The listing builds one solid part. Answer for the finished solid, in the listing's coordinates (mm). A direction names the side the tool comes from. Coordinates: 2 decimals unless noted, no trailing zeros. Loops run counter-clockwise (first coordinate to the right, second up) from the corner with the lowest first, then second, coordinate; pieces in that order, holes last. Notation, with made-up numbers: (56, 4) - (97, 4) arc R16 cw to (97, 25) - close; hole circle Ø5 at (37, -11.5). An arc over 180 degrees is marked (long way). Put each result on its own line as item: value.
```python
from build123d import *

# Parameters (mm, degrees)
SKETCH1_W                      = 150
SKETCH1_H                      = 26
BOSS_EXTRUDE1_DEPTH            = 8
SKETCH2_R                      = 1
CUT_EXTRUDE1_DEPTH             = 10
SKETCH3_R                      = 1
CUT_EXTRUDE2_DEPTH             = 10
SKETCH4_W                      = 65
SKETCH4_H                      = 30
BOSS_EXTRUDE2_DEPTH            = 8
FILLET1_R                      = 32
SKETCH5_W                      = 70
SKETCH5_H                      = 30
BOSS_EXTRUDE3_DEPTH            = 8
CBORE_FOR_M4_SHCS1_D           = 4.5
CBORE_FOR_M4_SHCS1_CBORE_D     = 8
CBORE_FOR_M4_SHCS1_CBORE_DEPTH = 4
SKETCH10_W                     = 18
SKETCH10_H                     = 17
BOSS_EXTRUDE4_DEPTH            = 8
FILLET2_R                      = 10
FILLET3_R                      = 2
FILLET4_R                      = 4
SKETCH11_R                     = 1.6
CUT_EXTRUDE3_DEPTH             = 82.172655494
CUT_EXTRUDE5_START             = -5.2
CUT_EXTRUDE5_DEPTH             = 2.4


with BuildPart() as part:
    # Sketch1 → Boss-Extrude1 (new body)
    with BuildSketch(Plane(origin=(0, 0, 0), x_dir=(1, 0, 0), z_dir=(0, 1, 0))):
        Rectangle(SKETCH1_W, SKETCH1_H)
    extrude(amount=BOSS_EXTRUDE1_DEPTH)

    # Sketch2 → Cut-Extrude1 (cut)
    with BuildSketch(Plane(origin=(0, 0, -13), x_dir=(-1, 0, 0), z_dir=(0, 0, -1))):
        with Locations((47.4, 3.5)):
            Circle(SKETCH2_R)
        with Locations((-49.4, 3.5)):
            Circle(SKETCH2_R)
    extrude(amount=-CUT_EXTRUDE1_DEPTH, mode=Mode.SUBTRACT)

    # Sketch3 → Cut-Extrude2 (cut)
    with BuildSketch(Plane.XY.offset(13)):
        with Locations((1, 3.5)):
            Circle(SKETCH3_R)
    extrude(amount=-CUT_EXTRUDE2_DEPTH, mode=Mode.SUBTRACT)

    # Sketch4 → Boss-Extrude2 (add)
    with BuildSketch(Plane(origin=(0, 0, 0), x_dir=(1, 0, 0), z_dir=(0, 1, 0))):
        with Locations((-42.5, -15)):
            Rectangle(SKETCH4_W, SKETCH4_H)
        with Locations((42.5, -15)):
            Rectangle(SKETCH4_W, SKETCH4_H)
    extrude(amount=BOSS_EXTRUDE2_DEPTH)

    # Fillet1
    fillet1_edges = [part.edges().sort_by_distance(p)[0] for p in [
        (-75, 4, 30),
        (75, 4, 30),
    ]]
    fillet(fillet1_edges, radius=FILLET1_R)

    # Sketch5 → Boss-Extrude3 (add)
    with BuildSketch(Plane(origin=(0, 0, 0), x_dir=(1, 0, 0), z_dir=(0, 1, 0))):
        with Locations((0, 15)):
            Rectangle(SKETCH5_W, SKETCH5_H)
    extrude(amount=BOSS_EXTRUDE3_DEPTH)

    # CBORE for M4 SHCS1 (through all)
    with Locations(Plane(origin=(0, 8, 0), x_dir=(1, 0, 0), z_dir=(0, 1, 0))):
        with Locations((-20, 25), (20, 25), (35, -25), (-35, -25)):
            CounterBoreHole(CBORE_FOR_M4_SHCS1_D / 2, CBORE_FOR_M4_SHCS1_CBORE_D / 2, CBORE_FOR_M4_SHCS1_CBORE_DEPTH)

    # Sketch10 → Boss-Extrude4 (add)
    with BuildSketch(Plane(origin=(0, 8, 0), x_dir=(1, 0, 0), z_dir=(0, 1, 0))):
        with Locations((-66, 21.5)):
            Rectangle(SKETCH10_W, SKETCH10_H)
        with Locations((66, 21.5)):
            Rectangle(SKETCH10_W, SKETCH10_H)
    extrude(amount=-BOSS_EXTRUDE4_DEPTH)

    # Fillet2
    fillet2_edges = [part.edges().sort_by_distance(p)[0] for p in [
        (-57, 4, -30),
        (57, 4, -30),
        (-10, 4, 30),
        (10, 4, 30),
        (-35, 4, -30),
        (35, 4, -30),
    ]]
    fillet(fillet2_edges, radius=FILLET2_R)

    # Fillet3
    fillet3_edges = [part.edges().sort_by_distance(p)[0] for p in [
        (-57, 4, -13),
        (57, 4, -13),
        (-10, 4, 13),
        (10, 4, 13),
        (-35, 4, -13),
        (35, 4, -13),
    ]]
    fillet(fillet3_edges, radius=FILLET3_R)

    # Fillet4
    fillet4_edges = [part.edges().sort_by_distance(p)[0] for p in [
        (-75, 4, -30),
        (75, 4, -30),
    ]]
    fillet(fillet4_edges, radius=FILLET4_R)

    # Sketch11 → Cut-Extrude3 (cut, through all)
    with BuildSketch(Plane(origin=(0, 8, 0), x_dir=(1, 0, 0), z_dir=(0, 1, 0))):
        with Locations(Location((-68, 25, 0), (0, 0, 270))):
            Circle(SKETCH11_R)
        with Locations(Location((-68, -7, 0), (0, 0, 270))):
            Circle(SKETCH11_R)
        with Locations(Location((0, 25, 0), (0, 0, 270))):
            Circle(SKETCH11_R)
        with Locations(Location((-22, -25, 0), (0, 0, 270))):
            Circle(SKETCH11_R)
        with Locations(Location((22, -25, 0), (0, 0, 270))):
            Circle(SKETCH11_R)
        with Locations(Location((68, -7, 0), (0, 0, 270))):
            Circle(SKETCH11_R)
        with Locations(Location((68, 25, 0), (0, 0, 270))):
            Circle(SKETCH11_R)
    extrude(amount=-CUT_EXTRUDE3_DEPTH, mode=Mode.SUBTRACT)

    # Sketch14 → Cut-Extrude5 (cut)
    with BuildSketch(Plane(origin=(0, 8, 0), x_dir=(1, 0, 0), z_dir=(0, 1, 0)).offset(CUT_EXTRUDE5_START)):
        Polygon((19.15, -26.645448267), (19.15, -29.963809512), (19.15, -31.088367393), (24.85, -31.088367393), (24.85, -30), (24.85, -26.645448267), (24.85, -23.354551733), (22, -21.709103466), (19.15, -23.354551733), align=None)
        Polygon((-70.85, 26.645448267), (-70.85, 23.354551733), (-68, 21.709103466), (-65.15, 23.354551733), (-65.15, 26.645448267), (-65.15, 32.162081996), (-70.85, 32.162081996), align=None)
        Polygon((-66.354551733, -9.85), (-64.709103466, -7), (-66.354551733, -4.15), (-69.645448267, -4.15), (-77.063489816, -4.15), (-77.063489816, -9.85), (-69.645448267, -9.85), align=None)
        Polygon((69.645448267, -4.15), (74.85540498, -4.15), (74.85540498, -9.85), (69.645448267, -9.85), (66.354551733, -9.85), (64.709103466, -7), (66.354551733, -4.15), align=None)
        Polygon((-19.15, -26.645448267), (-19.15, -23.354551733), (-22, -21.709103466), (-24.85, -23.354551733), (-24.85, -26.645448267), (-24.85, -31.723869118), (-19.15, -31.723869118), align=None)
        Polygon((65.15, 26.645448267), (65.15, 32.162081996), (70.85, 32.162081996), (70.85, 26.645448267), (70.85, 23.354551733), (68, 21.709103466), (65.15, 23.354551733), align=None)
        Polygon((-2.85, 26.645448267), (-2.85, 23.354551733), (0, 21.709103466), (2.85, 23.354551733), (2.85, 26.645448267), (2.85, 32.162081996), (-2.85, 32.162081996), align=None)
    extrude(amount=CUT_EXTRUDE5_DEPTH, mode=Mode.SUBTRACT)


solid = part.part
```
1) The part is cut by section B-B (x = 5). Give the vertices of the cut face in (y, z).
Found:
outline: (0, -30) - (8, -30) - (8, 13) - (0, 13) - close
2) Each of these flat-tipped pins is pushed along its axis until it touches: pin 1 (4 mm diameter, centred on x = -2.5, y = 2.5, fed in from +Z); pin 2 (9 mm diameter, centred on x = -35, z = 25, fed in from +Y); pin 3 (1.5 mm diameter, centred on y = 1, z = 11, fed in from -X); pin 4 (1.5 mm diameter, centred on x = 11, y = 5.5, fed in from +Z). Where does it stop, or does it pass through?
Found:
pin 1: stops at z = 13
pin 2: stops at y = 8
pin 3: stops at x = -72.56
pin 4: stops at z = 25.65
3) The part is cut by section A-A (z = 18.5). Give the vertices of the cut face in (x, y), and give its area (3 significant figures).
Found:
outline: (-67.57, 0) - (-10, 0) - (-10, 8) - (-67.57, 8) - close; (10, 0) - (67.57, 0) - (67.57, 8) - (10, 8) - close
area: 921 mm^2
4) Straight lines are drawn through the part: L1, parallel to X at y = 2.05, z = 25; L2, parallel to X at y = 6.2, z = 25; L3, parallel to X at y = 1.8, z = 7. For each, find the intervals that lie inside material, in ascending order. Write a range as [from, to].
Found:
L1: x = [-60.18, -37.25], [-32.75, -23.6], [-20.4, -11.34], [11.34, 20.4], [23.6, 32.75], [37.25, 60.18]
L2: x = [-60.18, -39], [-31, -23.6], [-20.4, -11.34], [11.34, 20.4], [23.6, 31], [39, 60.18]
L3: x = [-73.71, -69.6], [-66.4, 66.4], [69.6, 73.71]
5) For a pull along X with two mould halves and no side action, classify faces 4 (the face through (-68, 5.2, -27)), 5 (the face through (73.859, 3.944, -28.797)), 6 (the face through (-73.859, 3.944, -28.797)) as pulls with the +X half, pulls with the -X half, needs draft (parallel to the pull), parting line crosses it, or undercut.
Found:
face 4: undercut
face 5: pulls with the +X half
face 6: pulls with the -X half
6) For faces 1 (the face through (-59.85, 3.94, -26.99)), 2 (the face through (-20.521, 6.028, -28.966)), 3 (the face through (-22, 2.8, 27)), determine the directions among +Z, -Z, +X, -X, +Y, -Y from which every point of the face is accessible in a straight line to the end or side of a thin tool.
Found:
face 1: -Z, +Y, -Y
face 2: +Y
face 3: +Z
